Check sheet for the modelled part. Datum: model origin and axes. Units: mm. Face numbers are marked on the shaded views. Round coordinates to 2 decimals unless told otherwise and drop trailing zeros. Loops run counter-clockwise (first coordinate to the right, second up) from the corner with the lowest first, then second, coordinate; pieces in that order, holes last. Notation, with made-up numbers: (-22.5, 88) - (22.5, 88) arc R23 ccw to (22.5, 123) - close; hole circle Ø5 at (-21.5, 14.5). An arc over 180 degrees is marked (long way). Put each result on its own line as item: value.
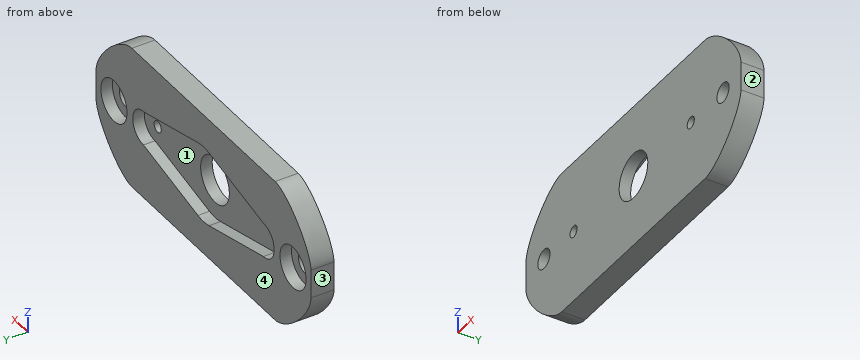
```python
from build123d import *

# Parameters (mm, degrees)
SKETCH1_W           = 60
SKETCH1_H           = 8
BOSS_EXTRUDE1_DEPTH = 25
SKETCH2_W           = 60
SKETCH2_H           = 2
CUT_EXTRUDE1_DEPTH  = 22
CUT_EXTRUDE2_DEPTH  = 2
SKETCH4_R           = 1
SKETCH4_R_2         = 4
CUT_EXTRUDE3_DEPTH  = 2.5
SKETCH5_R           = 1.7
CUT_EXTRUDE4_DEPTH  = 9
FILLET2_SIZE        = 10
SKETCH6_R           = 3
CUT_EXTRUDE5_DEPTH  = 4.5
CUT_EXTRUDE6_DEPTH  = 1
SKETCH8_R           = 3.65
CUT_EXTRUDE7_DEPTH  = 2
SKETCH10_W          = 50
SKETCH10_H          = 4
CUT_EXTRUDE8_DEPTH  = 61


with BuildPart() as part:
    # Sketch1 → Boss-Extrude1 (new body)
    with BuildSketch(Plane.XY):
        with Locations((9.92851316, -6.03519833)):
            Rectangle(SKETCH1_W, SKETCH1_H)
    extrude(amount=BOSS_EXTRUDE1_DEPTH)

    # Sketch2 → Cut-Extrude1 (cut)
    with BuildSketch(Plane.XY.offset(25)):
        with Locations((9.92851316, -7.03519833)):
            Rectangle(SKETCH2_W, SKETCH2_H)
    extrude(amount=-CUT_EXTRUDE1_DEPTH, mode=Mode.SUBTRACT)

    # Sketch3 → Cut-Extrude2 (cut)
    with BuildSketch(Plane(origin=(0, -2.03519833, 0), x_dir=(1, 0, 0), z_dir=(0, 1, 0))):
        with BuildLine():
            Line((26.67851316, -9.5), (11.471726674, -5.928775453))
            ThreePointArc((11.471726674, -5.928775453), (9.92851316, -5.75), (8.385299646, -5.928775453))
            Line((8.385299646, -5.928775453), (-6.82148684, -9.5))
            ThreePointArc((-6.82148684, -9.5), (-9.821486841, -12.5), (-6.82148684, -15.5))
            Line((-6.82148684, -15.5), (8.385299646, -19.071224547))
            ThreePointArc((8.385299646, -19.071224547), (9.92851316, -19.25), (11.471726674, -19.071224547))
            Line((11.471726674, -19.071224547), (26.67851316, -15.5))
            ThreePointArc((26.67851316, -15.5), (29.67851316, -12.5), (26.67851316, -9.5))
        make_face()
    extrude(amount=-CUT_EXTRUDE2_DEPTH, mode=Mode.SUBTRACT)

    # Sketch4 → Cut-Extrude3 (cut)
    with BuildSketch(Plane(origin=(0, -4.03519833, 0), x_dir=(1, 0, 0), z_dir=(0, 1, 0))):
        with Locations(Location((-6.796927173, -12.5, 0), (0, 0, 270))):
            Circle(SKETCH4_R)
        with Locations(Location((9.92851316, -12.5, 0), (0, 0, 270))):
            Circle(SKETCH4_R_2)
        with Locations(Location((25.92851316, -12.5, 0), (0, 0, 270))):
            Circle(SKETCH4_R)
    extrude(amount=-CUT_EXTRUDE3_DEPTH, mode=Mode.SUBTRACT)

    # Sketch5 → Cut-Extrude4 (cut)
    with BuildSketch(Plane(origin=(0, -2.03519833, 0), x_dir=(1, 0, 0), z_dir=(0, 1, 0))):
        with Locations(Location((34.92851316, -12.5, 0), (0, 0, 270))):
            Circle(SKETCH5_R)
        with Locations(Location((-15.07148684, -12.5, 0), (0, 0, 270))):
            Circle(SKETCH5_R)
    extrude(amount=-CUT_EXTRUDE4_DEPTH, mode=Mode.SUBTRACT)

    # Fillet2
    # a fillet whose section is not a circle: 10 mm, written as the material it takes off along each edge
    with BuildSketch(Plane(origin=(-20.07148684, -31.03519833, 25), x_dir=(0, 0, -1), z_dir=(0, 1, 0))) as fillet2_piece_1:
        with BuildLine():
            Bezier((FILLET2_SIZE, 0), (0, 0), (0, -FILLET2_SIZE), weights=[1, 0.353553391, 1])
            Line((0, -FILLET2_SIZE), (0, 0))
            Line((0, 0), (FILLET2_SIZE, 0))
        make_face()
    extrude(amount=54, mode=Mode.SUBTRACT)
    with BuildSketch(Plane(origin=(-20.07148684, -35.03519833, 25), x_dir=(0, 0, -1), z_dir=(0, 1, 0)), Plane(origin=(39.92851316, 16.96480167, 25), x_dir=(0, 0, -1), z_dir=(0, -1, 0))) as fillet2_piece_2:
        with BuildLine():
            Bezier((FILLET2_SIZE, 0), (0, 0), (0, -FILLET2_SIZE), weights=[1, 0.353553391, 1])
            Line((0, -FILLET2_SIZE), (0, 0))
            Line((0, 0), (FILLET2_SIZE, 0))
        make_face()
    extrude(amount=52, mode=Mode.SUBTRACT)
    with BuildSketch(Plane(origin=(39.92851316, 22.96480167, 25), x_dir=(-1, 0, 0), z_dir=(0, -1, 0))) as fillet2_piece_3:
        with BuildLine():
            Bezier((FILLET2_SIZE, 0), (0, 0), (0, FILLET2_SIZE), weights=[1, 0.353553391, 1])
            Line((0, FILLET2_SIZE), (0, 0))
            Line((0, 0), (FILLET2_SIZE, 0))
        make_face()
    extrude(amount=54, mode=Mode.SUBTRACT)
    with BuildSketch(Plane(origin=(39.92851316, 22.96480167, 0), x_dir=(-1, 0, 0), z_dir=(0, -1, 0))) as fillet2_piece_4:
        with BuildLine():
            Bezier((FILLET2_SIZE, 0), (0, 0), (0, -FILLET2_SIZE), weights=[1, 0.353553391, 1])
            Line((0, -FILLET2_SIZE), (0, 0))
            Line((0, 0), (FILLET2_SIZE, 0))
        make_face()
    extrude(amount=58, mode=Mode.SUBTRACT)
    with BuildSketch(Plane(origin=(-20.07148684, -35.03519833, 0), x_dir=(0, 0, 1), z_dir=(0, 1, 0))) as fillet2_piece_5:
        with BuildLine():
            Bezier((FILLET2_SIZE, 0), (0, 0), (0, FILLET2_SIZE), weights=[1, 0.353553391, 1])
            Line((0, FILLET2_SIZE), (0, 0))
            Line((0, 0), (FILLET2_SIZE, 0))
        make_face()
    extrude(amount=58, mode=Mode.SUBTRACT)

    # Sketch6 → Cut-Extrude5 (cut)
    with BuildSketch(Plane(origin=(0, -8.03519833, 0), x_dir=(1, 0, 0), z_dir=(0, 1, 0))):
        with Locations(Location((9.92851316, -12.5, 0), (0, 0, 270))):
            Circle(SKETCH6_R)
    extrude(amount=-CUT_EXTRUDE5_DEPTH, mode=Mode.SUBTRACT)

    # Sketch7 → Cut-Extrude6 (cut)
    with BuildSketch(Plane(origin=(0, -10.03519833, 0), x_dir=(-1, 0, 0), z_dir=(0, -1, 0))):
        Polygon((-35.683884991, -9.237677709), (-38.131453055, -11.52301005), (-37.376081224, -14.785332341), (-34.173141329, -15.762322291), (-31.725573265, -13.47698995), (-32.480945096, -10.214667659), align=None)
        Polygon((12.105656047, -10.945271393), (12.242136974, -14.291120506), (15.207967766, -15.845849113), (18.037317633, -14.054728607), (17.900836706, -10.708879494), (14.935005914, -9.154150887), align=None)
    extrude(amount=-CUT_EXTRUDE6_DEPTH, mode=Mode.SUBTRACT)

    # Sketch8 → Cut-Extrude7 (cut)
    with BuildSketch(Plane(origin=(0, -2.03519833, 0), x_dir=(1, 0, 0), z_dir=(0, 1, 0))):
        with Locations(Location((-15.07148684, -12.5, 0), (0, 0, 270))):
            Circle(SKETCH8_R)
        with Locations(Location((34.92851316, -12.5, 0), (0, 0, 270))):
            Circle(SKETCH8_R)
    extrude(amount=-CUT_EXTRUDE7_DEPTH, mode=Mode.SUBTRACT)

    # Sketch10 → Cut-Extrude8 (cut)
    with BuildSketch(Plane.ZY.offset(20.07148684)):
        with Locations((25, -8.03519833)):
            Rectangle(SKETCH10_W, SKETCH10_H)
    extrude(amount=-CUT_EXTRUDE8_DEPTH, mode=Mode.SUBTRACT)


solid = part.part
```
Item 1: Section check B-B on z = 12.5. Count the separate pieces of the cut face and the enclosed holes in it, then the cut area to 3 significant figures.
Filled sheet:
separate pieces: 6
enclosed holes: 0
area: 94.2 mm²
Item 2: Section check A-A on x = 21. Enter the section's corners in (y, z), then the cut area to 3 significant figures.
Filled sheet:
outline: (-6.04, 0) - (-2.04, 0) - (-2.04, 8.17) - (-4.04, 8.17) - (-4.04, 16.83) - (-2.04, 16.83) - (-2.04, 25) - (-6.04, 25) - close
area: 82.7 mm²
Item 3: Thickness scan on line 1 (X direction, y = -4.9, z = 12.5); line 2 (X direction, y = -2.8, z = 12.5); line 3 (Y direction, x = 32.5, z = 14.75). Record the ranges inside material, lowest first. Write a range as from..to.
Filled sheet:
line 1: -20.07..-16.77, -13.37..-7.8, -5.8..5.93, 13.93..24.93, 26.93..33.23, 36.63..39.93
line 2: -20.07..-18.72, -11.42..-9.82, 29.68..31.28, 38.58..39.93
line 3: -6.04..-4.04
Item 4: Section check D-D on x = 2. Enter the section's corners in (y, z), then the cut area to 3 significant figures.
Filled sheet:
outline: (-6.04, 0) - (-2.04, 0) - (-2.04, 7.43) - (-4.04, 7.43) - (-4.04, 17.57) - (-2.04, 17.57) - (-2.04, 25) - (-6.04, 25) - close
area: 79.7 mm²
Item 5: Release check for a two-part mould opening along X. For the marked faces 1, 2, 3 and 4 record: +X half, -X half, draft (parallel to the pull), parting line (faces both ways), or undercut.
Filled sheet:
face 1: undercut
face 2: +X half
face 3: -X half
face 4: draft
Item 6: Go/stop test with flat-tipped pins: pin 1 (2.5 mm diameter, centred on x = -6.8, z = 12.5, fed in from +Y); pin 2 (1.2 mm diameter, centred on x = 25.93, z = 12.5, fed in from +Y); pin 3 (2 mm diameter, centred on y = -5.5, z = 20, fed in from +X). Record where each tip stops, or that it passes through.
Filled sheet:
pin 1: y = -4.04
pin 2: through
pin 3: x = 38.2
